Build history of the part. All positions in model axes, mm. A direction names the side the tool comes from. Give positions to 0.01 mm unless a question says otherwise; leave off trailing zeros. Write each loop counter-clockwise with the first axis right and the second up, starting at its lowest first coordinate (ties: lowest second). Pieces come first, ordered by that corner, then holes. Notation, with made-up numbers: (13, 23) -> (37, 23) arc R19 cw to (37, 30) -> close; hole circle Ø1 at (8.5, 84). An arc over 180 degrees is marked (long way). Put each result on its own line as item: value.
from build123d import *

# Parameters (mm, degrees)
BOSS_EXTRUDE1_DEPTH        = 7
BOSS_EXTRUDE2_DEPTH        = 2
BOSS_EXTRUDE3_DEPTH        = 2
BOSS_EXTRUDE4_START        = 2
BOSS_EXTRUDE4_DEPTH        = 1.5
WIRE_START                 = -3
SKETCH3_R                  = 1.75
WIRE_AND_TUBE_CANALS_DEPTH = 8.5
SKETCH5_R                  = 0.8
SKETCH5_R_2                = 0.799999999
SCREW_HOLES_DEPTH          = 8.0000001
CUT_EXTRUDE1_START         = 4
CUT_EXTRUDE1_DEPTH         = 3


with BuildPart() as part:
    # Sketch1 → Boss-Extrude1 (new body)
    with BuildSketch(Plane.XY):
        with BuildLine():
            Line((13.246912191, -20.732193563), (3.347417254, -30.6316885))
            Line((3.347417254, -30.6316885), (0, -27.284271246))
            Line((0, -27.284271246), (0, -0.797958973))
            ThreePointArc((0, -0.797958973), (9.999999999, -5), (19.999999998, -0.797958971))
            Line((19.999999998, -0.797958971), (19.999999998, -19))
            Line((19.999999998, -19), (22.085746954, -21.085746956))
            Line((22.085746954, -21.085746956), (17.843106269, -25.328387641))
            Line((17.843106269, -25.328387641), (13.246912191, -20.732193563))
        make_face()
        Polygon((1, -15.5), (1, -26.870057685), (3.347417253, -29.217474938), (15.999999998, -16.564892192), (15.999999998, -11.5), (4, -11.5), (4, -15.5), align=None, mode=Mode.SUBTRACT)
    extrude(amount=BOSS_EXTRUDE1_DEPTH)

    # Sketch6 → Boss-Extrude2 (add)
    with BuildSketch(Plane.XY):
        Polygon((1, -11.5), (3, -11.5), (3, -26.87005769), (17, -12.87005769), (17, -11.500000008), (19, -11.500000008), (19, -18.000000005), (17.843106267, -16.843106272), (14.307572361, -20.378640178), (13.246912189, -19.317980006), (3.347417253, -29.217474943), (1, -26.87005769), align=None)
    extrude(amount=BOSS_EXTRUDE2_DEPTH)

    # Sketch8 → Boss-Extrude3 (add)
    with BuildSketch(Plane.XY):
        with BuildLine():
            Line((10, -11.5), (12.5, -11.5))
            Line((12.5, -11.5), (12.5, 9))
            ThreePointArc((12.5, 9), (10, 11.5), (7.5, 9))
            Line((7.5, 9), (7.5, -11.5))
            Line((7.5, -11.5), (10, -11.5))
        make_face()
    extrude(amount=BOSS_EXTRUDE3_DEPTH)

    # Sketch9 → Boss-Extrude4 (add)
    with BuildSketch(Plane.XY.offset(BOSS_EXTRUDE4_START)):
        with BuildLine():
            Line((8.397853003, 9.925), (11.602146997, 9.925))
            ThreePointArc((11.602146997, 9.925), (10, 7.15), (8.397853003, 9.925))
        make_face()
    extrude(amount=BOSS_EXTRUDE4_DEPTH)

    # Sketch3 → Wire and Tube Canals (cut)
    with BuildSketch(Plane(origin=(0, 0, 0), x_dir=(1, 0, 0), z_dir=(0, 1, 0)).offset(WIRE_START)):
        with Locations((6, -7)):
            Circle(SKETCH3_R)
        with Locations((14, -7)):
            Circle(SKETCH3_R)
        Polygon((6, -6), (8, -6), (8, -5), (12, -5), (12, -6), (14, -6), (14, -7), (6, -7), align=None)
    extrude(amount=-WIRE_AND_TUBE_CANALS_DEPTH, mode=Mode.SUBTRACT)

    # Sketch5 → Screw Holes (cut, through all)
    with BuildSketch(Plane.XY):
        with Locations((2, -6.5)):
            Circle(SKETCH5_R)
        with Locations((2, -9.5)):
            Circle(SKETCH5_R)
        with Locations((18, -9.5)):
            Circle(SKETCH5_R)
        with Locations((18, -6.5)):
            Circle(SKETCH5_R)
        with Locations((18.90376644, -22.146407127)):
            Circle(SKETCH5_R_2)
        with Locations((16.782446096, -20.025086783)):
            Circle(SKETCH5_R_2)
        with Locations((2, -13.5)):
            Circle(SKETCH5_R)
        with Locations((18, -13.5)):
            Circle(SKETCH5_R)
    extrude(amount=SCREW_HOLES_DEPTH, mode=Mode.SUBTRACT)

    # Sketch10 → Cut-Extrude1 (cut)
    with BuildSketch(Plane.XY.offset(CUT_EXTRUDE1_START)):
        Polygon((17.843106269, -25.328387641), (22.085746954, -21.085746956), (15.721785923, -14.721785925), (11.479145238, -18.96442661), align=None)
    extrude(amount=CUT_EXTRUDE1_DEPTH, mode=Mode.SUBTRACT)


solid = part.part
1) Pin check, flat tips, straight feed: pin 1 (2.5 mm diameter, centred on x = 2, y = -6.5, fed in from +Z); pin 2 (0.6 mm diameter, centred on y = 4, z = 1, fed in from -X); pin 3 (5 mm diameter, centred on x = 19.5, y = -21.5, fed in from +Z); pin 4 (1.6 mm diameter, centred on y = 0.5, z = 1, fed in from +X). Stop position of each tip, or through.
Filled sheet:
pin 1: z = 7
pin 2: x = 7.5
pin 3: z = 4
pin 4: x = 12.5
2) Pull direction X, two halves, no side cores. Call faces 1 (the flat face through (10, 9.925, 3)), 2 (the cylindrical face through (10.1, 11.5, 1)), 3 (the cylindrical face through (1.896, -8.707, 3.451)): released by +X, released by -X, zero draft, split by the parting line, or undercut.
Filled sheet:
face 1: zero draft
face 2: split by the parting line
face 3: undercut
3) Tool access for faces 4 (the flat face through (10, 3, 2)), 5 (the cylindrical face through (14.55, -7.58, 5.34)), 6 (the flat face through (8.37, -25.61, 3.45)), 7 (the flat face through (10, -11.5, 3)): list every direction of +Z, -Z, +X, -X, +Y, -Y with a clear straight run to the whole face (end or side of a thin tool).
Filled sheet:
face 4: +Z
face 5: +Z, +Y
face 6: +Z, -Z, -Y
face 7: +Z, -Z
4) Slice it at B-B (x = 15.25). Write the cut outline in (y, z), plus the area to 3 significant figures.
Filled sheet:
outline: (-22.74, 0) -> (-14.62, 0) -> (-14.62, 2) -> (-17.31, 2) -> (-17.31, 4) -> (-22.74, 4) -> close; (-11.5, 0) -> (-3.98, 0) -> (-3.98, 5.78) -> (-11.5, 5.78) -> close
area: 70.5 mm2
5) Slice it at C-C (x = 2). Write the cut outline in (y, z).
Filled sheet:
outline: (-29.28, 0) -> (-14.3, 0) -> (-14.3, 7) -> (-15.5, 7) -> (-15.5, 2) -> (-27.87, 2) -> (-27.87, 7) -> (-29.28, 7) -> close; (-12.7, 0) -> (-10.3, 0) -> (-10.3, 7) -> (-12.7, 7) -> close; (-8.7, 0) -> (-7.3, 0) -> (-7.3, 7) -> (-8.7, 7) -> close; (-5.7, 0) -> (-2.49, 0) -> (-2.49, 7) -> (-5.7, 7) -> close
6) Slice it at A-A (y = -6.5). Write the cut outline in (x, z).
Filled sheet:
outline: (0, 0) -> (1.2, 0) -> (1.2, 7) -> (0, 7) -> close; (2.8, 0) -> (17.2, 0) -> (17.2, 7) -> (15.75, 7) arc R1.75 cw to (12.56, 6) -> (12, 6) -> (12, 5) -> (8, 5) -> (8, 6) -> (7.44, 6) arc R1.75 cw to (4.25, 7) -> (2.8, 7) -> close; (18.8, 0) -> (20, 0) -> (20, 7) -> (18.8, 7) -> close
7) Slice it at D-D (x = 6.5). Write the cut outline in (y, z).
Filled sheet:
outline: (-27.48, 0) -> (-23.37, 0) -> (-23.37, 2) -> (-26.06, 2) -> (-26.06, 7) -> (-27.48, 7) -> close; (-11.5, 0) -> (-4.56, 0) -> (-4.56, 5.32) -> (-11.5, 5.32) -> close
8) Wall check: L1, parallel to X at y = -13.5, z = 3; L2, parallel to X at y = -9, z = 6.75; L3, parallel to Y at x = 18, z = 3. Give the ranges that are in metal, low to high.
Filled sheet:
L1: 0 to 1.2, 2.8 to 4, 16 to 17.2, 18.8 to 20
L2: 0 to 1.38, 2.62 to 4.27, 15.73 to 17.38, 18.62 to 20
L3: -25.17 to -14.3, -12.7 to -10.3, -8.7 to -7.3, -5.7 to -2.49
